Work out the finished part from the listing and answer in its coordinate system (mm). A direction names the side the tool comes from. Coordinates: 2 decimals unless noted, no trailing zeros. Write each loop counter-clockwise with the first axis right and the second up, starting at its lowest first coordinate (ties: lowest second). Pieces come first, ordered by that corner, then holes. Notation, with made-up numbers: (-4, -5) - (10, -5) arc R23 ccw to (10, 20) - close; hole circle Ø8 at (18, 3). An arc over 180 degrees is marked (long way). Use a Markdown table: item, result. Add a question column.
(1) For a pull along Y with two mould halves and no side action, classify faces 5 (the face through (-0.1, -6.2, 0)), 6 (the face through (6.92, 0.3, 5.95)), 7 (the face through (-1.08, -4.88, 4.8)), 8 (the face through (-3.229, -6.468, 1.785)) as released by +Y, released by -Y, zero draft, split by the parting line, or undercut.
(2) Given pin 1 Ø1 at (y, z) = (-6, 3.5) entering from +X; pin 2 Ø1 at (x, z) = (7.5, 2.5) entering from -Y, each flat-ended and moving along its own axis, determine where each tip first touches the part or whether it passes through.
(3) The part is cut by section A-A, the plane z = 8. Give the vertices of the cut face in (x, y), then the cut area to 3 significant figures.
(4) A tool of negligible diameter and unlimited length cuts with its end or side. For faces 1 (the face through (3.723, -5.843, 5.951)), 2 (the face through (-4.3, -7, 1.5)), 3 (the face through (-6.92, -0.3, 5.95)), 4 (the face through (-3.723, 5.843, 5.951)), from which of +Z, -Z, +X, -X, +Y, -Y can it reach the whole face along a straight path? Write none if from no direction.
(5) Find the intervals of material crossed by line 1 (Y direction, x = 0, z = 6); line 2 (Y direction, x = -4.25, z = 8.25); line 3 (Z direction, x = -8, y = 3), in increasing order. Write a range as from..to.
from build123d import *

# Parameters (mm, degrees)
SKETCH1_R           = 10
BOSS_EXTRUDE2_DEPTH = 1.5
FILLET1_R           = 0.5
BOSS_EXTRUDE3_DEPTH = 8
FILLET2_R           = 1
SKETCH5_R           = 5
CUT_EXTRUDE1_DEPTH  = 18.036725155
FILLET3_R           = 1


with BuildPart() as part:
    # Sketch1 → Boss-Extrude2 (new body)
    with BuildSketch(Plane.XY):
        Circle(SKETCH1_R)
    extrude(amount=BOSS_EXTRUDE2_DEPTH)

    # Fillet1
    fillet1_edges = [part.edges().sort_by_distance(p)[0] for p in [
        (-10, 0, 0),
        (-10, 0, 1.5),
    ]]
    fillet(fillet1_edges, radius=FILLET1_R)

    # Sketch3 → Boss-Extrude3 (add)
    with BuildSketch(Plane.XY.offset(1.5)):
        Polygon((-7.125875884, 3.636192085), (-6.711972661, -4.353093498), (0.413903224, -7.989285583), (7.125875884, -3.636192085), (6.711972661, 4.353093498), (-0.413903224, 7.989285583), align=None)
    extrude(amount=BOSS_EXTRUDE3_DEPTH)

    # Fillet2
    fillet2_edges = [part.edges().sort_by_distance(p)[0] for p in [
        (-3.769889554, 5.812738834, 1.5),
        (-6.918924273, -0.358450706, 1.5),
        (-3.149034719, -6.17118954, 1.5),
        (3.769889554, -5.812738834, 1.5),
        (6.918924273, 0.358450706, 1.5),
        (3.149034719, 6.17118954, 1.5),
    ]]
    fillet(fillet2_edges, radius=FILLET2_R)

    # Sketch5 → Cut-Extrude1 (cut, through all)
    with BuildSketch(Plane.XY.offset(9.5)):
        Circle(SKETCH5_R)
    extrude(amount=-CUT_EXTRUDE1_DEPTH, mode=Mode.SUBTRACT)

    # Fillet3
    fillet3_edges = [part.edges().sort_by_distance(p)[0] for p in [
        (-5, 0, 0),
        (-5, 0, 9.5),
    ]]
    fillet(fillet3_edges, radius=FILLET3_R)


solid = part.part
Model answer:
| question | item | result |
|---|---|---|
| 1 | face 5 | zero draft |
| 1 | face 6 | released by +Y |
| 1 | face 7 | undercut |
| 1 | face 8 | released by -Y |
| 2 | pin 1 | x = 4.25 |
| 2 | pin 2 | y = -3.72 |
| 3 | outline | (-7.13, 3.64) - (-6.71, -4.35) - (0.41, -7.99) - (7.13, -3.64) - (6.71, 4.35) - (-0.41, 7.99) - close; hole circle Ø10 at (0, 0) |
| 3 | area | 87.7 mm^2 |
| 4 | face 1 | +Z, +X, -Y |
| 4 | face 2 | +Z |
| 4 | face 3 | +Z, -X, -Y |
| 4 | face 4 | +Z, -X, +Y |
| 5 | line 1 | -7.78..-5, 5..7.78 |
| 5 | line 2 | -5.61..-2.63, 2.63..5.5 |
| 5 | line 3 | 0..1.5 |
